For this review, use the dimensioned drawing (mm, ordinates from the lowest corner) and the shaded views. Coordinates: 2 decimals unless noted, no trailing zeros. Loops run counter-clockwise (first coordinate to the right, second up) from the corner with the lowest first, then second, coordinate; pieces in that order, holes last.
1. Take a section at D-D, the plane x = 14. State the section outline as (y, z) points.
2. Clearance check with a flat-ended pin moving along its axis: P1, Ø1.8, axis at x = 18, y = 6, coming from the +Z side. State where the tip first meets the part, or that it passes through.
3. Take a section at B-B, the plane y = 22. State the section outline as (x, z) points, then the cut area to 3 significant figures.
4. Take a section at C-C, the plane y = 18. State the section outline as (x, z) points, then the cut area to 3 significant figures.
5. Take a section at A-A, the plane x = 18. State the section outline as (y, z) points.
6. To check wall thickness, follow probe 1 along Y at (x, z) = (14.75, 0.7); probe 2 along X at (y, z) = (5.25, 2.1); probe 3 along Y at (x, z) = (6, 0.55). State the ranges of each line that lie inside material, in increasing order.
7. Mouldability with a two-part tool opening along Y and no side actions: class the marked faces 1, 2 and 3 as pulls with the +Y half, pulls with the -Y half, needs draft (parallel to the pull), parting line crosses it, or undercut.
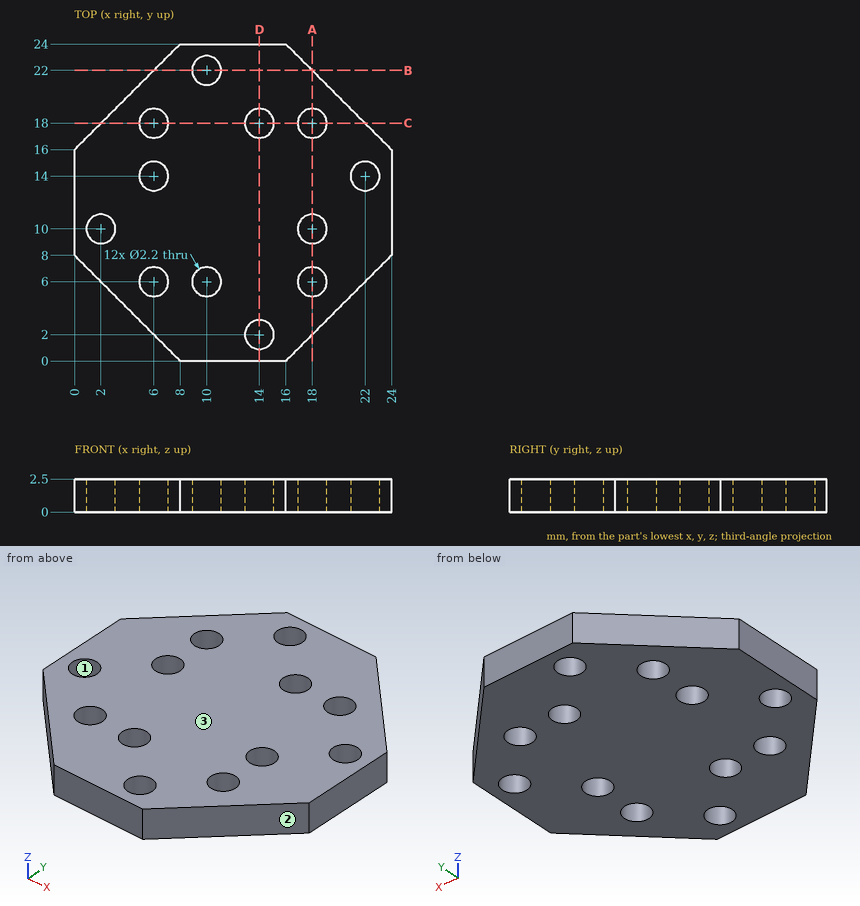
Results list:
1. outline: (0, 0) - (0.9, 0) - (0.9, 2.5) - (0, 2.5) - close; (3.1, 0) - (16.9, 0) - (16.9, 2.5) - (3.1, 2.5) - close; (19.1, 0) - (24, 0) - (24, 2.5) - (19.1, 2.5) - close
2. P1: passes through
3. outline: (6, 0) - (8.9, 0) - (8.9, 2.5) - (6, 2.5) - close; (11.1, 0) - (18, 0) - (18, 2.5) - (11.1, 2.5) - close
3. area: 24.5 mm2
4. outline: (2, 0) - (4.9, 0) - (4.9, 2.5) - (2, 2.5) - close; (7.1, 0) - (12.9, 0) - (12.9, 2.5) - (7.1, 2.5) - close; (15.1, 0) - (16.9, 0) - (16.9, 2.5) - (15.1, 2.5) - close; (19.1, 0) - (22, 0) - (22, 2.5) - (19.1, 2.5) - close
4. area: 33.5 mm2
5. outline: (2, 0) - (4.9, 0) - (4.9, 2.5) - (2, 2.5) - close; (7.1, 0) - (8.9, 0) - (8.9, 2.5) - (7.1, 2.5) - close; (11.1, 0) - (16.9, 0) - (16.9, 2.5) - (11.1, 2.5) - close; (19.1, 0) - (22, 0) - (22, 2.5) - (19.1, 2.5) - close
6. probe 1: y = 0 to 1.2, 2.8 to 17.2, 18.8 to 24
6. probe 2: x = 2.75 to 5.2, 6.8 to 9.2, 10.8 to 17.2, 18.8 to 21.25
6. probe 3: y = 2 to 4.9, 7.1 to 12.9, 15.1 to 16.9, 19.1 to 22
7. face 1: undercut
7. face 2: pulls with the -Y half
7. face 3: needs draft
